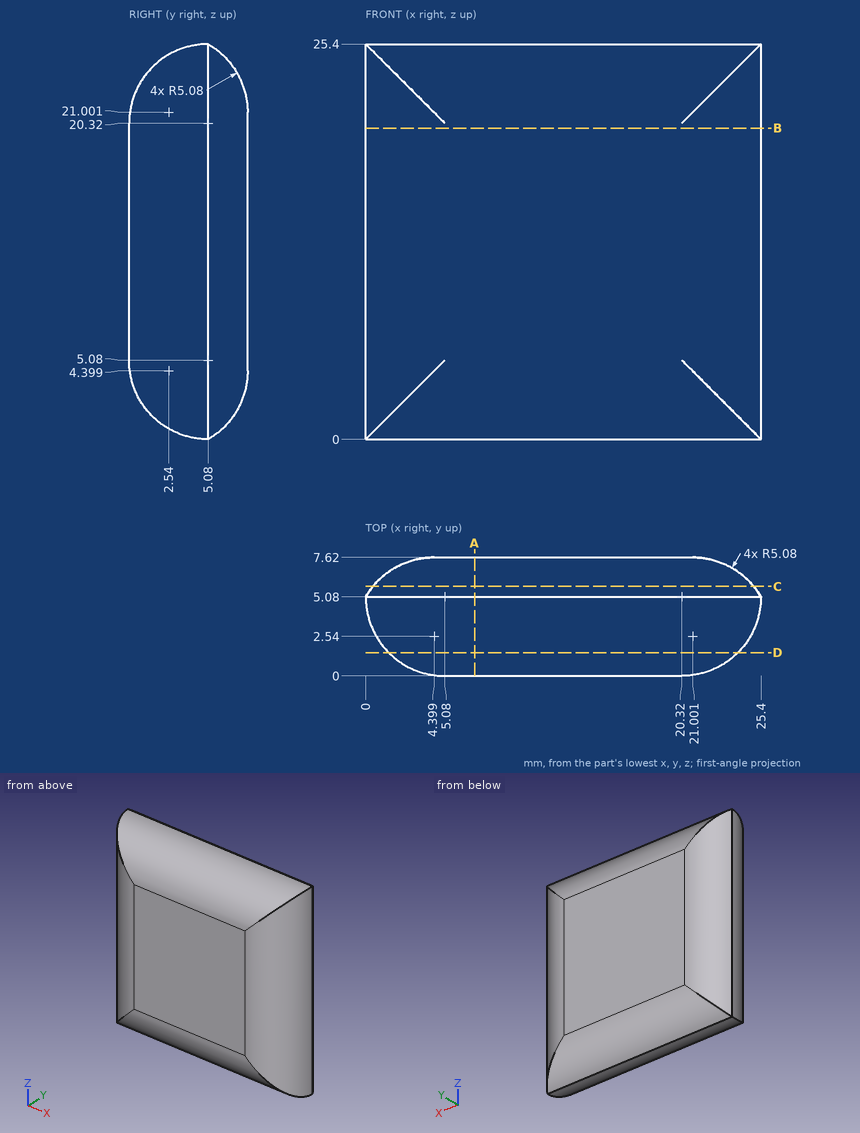
Can you work these out from the drawing? Everything is in mm from the part's minimum corner. Round coordinates to 2 decimals unless told otherwise and drop trailing zeros. Order: outer loops, then holes, each group sorted by start corner. A loop starts at its lowest first (then second) coordinate and runs counter-clockwise, first axis right, second up. Notation, with made-up numbers: (30, 72.5) -> (75, 72.5) arc R8 cw to (75, 87.5) -> close; hole circle Ø7 at (-25.5, 78.25). An arc over 180 degrees is marked (long way). Return JSON: item names as keys, results as strings. Group by question number.
1. If we section it at D-D, the plane y = 1.5: Write out the boundary of the cut face in (x, z), then the cut area to 3 significant figures.
2. Will these pins go through, and if not, where does the flat tip stop? pin 1 (2 mm diameter, centred on y = 5.5, z = 5, fed in from -X); pin 2 (4 mm diameter, centred on x = 19, y = 2, fed in from +Z).
3. I need wall thicknesses on line 1 (X direction, y = 2.75, z = 13.75) (1 decimal); line 2 (X direction, y = 5.5, z = 13.5); line 3 (Y direction, x = 23.75, z = 17) (1 decimal). Which ranges of each line are inside material? Lowest first, please. Write a range as [from, to].
4. If we section it at C-C, the plane y = 5.75: Write out the boundary of the cut face in (x, z).
5. If we section it at B-B, the plane z = 20: Write out the boundary of the cut face in (x, y).
6. If we section it at A-A, the plane x = 7: Write out the boundary of the cut face in (y, z), then the cut area to 3 significant figures.
Output values:
{
 "1": {"outline": "(1.48, 1.48) -> (23.92, 1.48) -> (23.92, 23.92) -> (1.48, 23.92) -> close", "area": "504 mm²"},
 "2": {"pin 1": "x = 0", "pin 2": "z = 25.28"},
 "3": {"line 1": "[0.6, 24.8]", "line 2": "[0.27, 25.13]", "line 3": "[1.3, 6.8]"},
 "4": {"outline": "(0.46, 0.46) -> (24.94, 0.46) -> (24.94, 24.94) -> (0.46, 24.94) -> close"},
 "5": {"outline": "(0, 5.08) arc R5.08 ccw to (5.08, 0) -> (20.32, 0) arc R5.08 ccw to (25.4, 5.08) arc R5.08 ccw to (21, 7.62) -> (4.4, 7.62) arc R5.08 ccw to start"},
 "6": {"outline": "(0, 5.08) arc R5.08 ccw to (5.08, 0) arc R5.08 ccw to (7.62, 4.4) -> (7.62, 21) arc R5.08 ccw to (5.08, 25.4) arc R5.08 ccw to (0, 20.32) -> close", "area": "176 mm²"}
}
